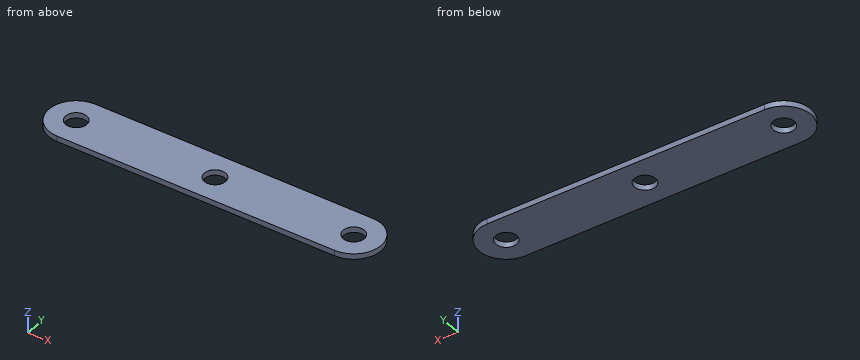
```python
from build123d import *

# Parameters (mm, degrees)
BOSS_EXTRUDE1_DEPTH = 4
CUT_EXTRUDE1_REACH  = 6
SKETCH2_R           = 7.75
CUT_EXTRUDE2_REACH  = 6
SKETCH3_R           = 7.75


with BuildPart() as part:
    # Sketch1 → Boss-Extrude1 (new body)
    with BuildSketch(Plane.XY):
        with BuildLine():
            Line((0, 20), (204, 20))
            ThreePointArc((204, 20), (224, 0), (204, -20))
            Line((204, -20), (0, -20))
            ThreePointArc((0, -20), (-20, 0), (0, 20))
        make_face()
    extrude(amount=BOSS_EXTRUDE1_DEPTH)

    # Sketch2 → Cut-Extrude1 (cut, up to next)
    with BuildSketch(Plane.XY.offset(4), mode=Mode.PRIVATE) as cut_extrude1_sk1:
        Circle(SKETCH2_R)
    cut_extrude1_tool1 = extrude(cut_extrude1_sk1.sketch, amount=-CUT_EXTRUDE1_REACH, mode=Mode.PRIVATE) & part.part
    add(cut_extrude1_tool1.solids().sort_by_distance((0, 0, 4))[0], mode=Mode.SUBTRACT)
    # Sketch2 → Cut-Extrude1 (cut, up to next)
    with BuildSketch(Plane.XY.offset(4), mode=Mode.PRIVATE) as cut_extrude1_sk2:
        with Locations((204, 0)):
            Circle(SKETCH2_R)
    cut_extrude1_tool2 = extrude(cut_extrude1_sk2.sketch, amount=-CUT_EXTRUDE1_REACH, mode=Mode.PRIVATE) & part.part
    add(cut_extrude1_tool2.solids().sort_by_distance((204, 0, 4))[0], mode=Mode.SUBTRACT)

    # Sketch3 → Cut-Extrude2 (cut, up to next)
    with BuildSketch(Plane.XY.offset(4), mode=Mode.PRIVATE) as cut_extrude2_sk1:
        with Locations((102, 0)):
            Circle(SKETCH3_R)
    cut_extrude2_tool1 = extrude(cut_extrude2_sk1.sketch, amount=-CUT_EXTRUDE2_REACH, mode=Mode.PRIVATE) & part.part
    add(cut_extrude2_tool1.solids().sort_by_distance((102, 0, 4))[0], mode=Mode.SUBTRACT)


solid = part.part
```
Geometry check sheet. Reference: the model listing, model coordinates, mm. Give positions to 0.01 mm unless a question says otherwise; leave off trailing zeros. Order: outer loops, then holes, each group sorted by start corner. A loop starts at its lowest first (then second) coordinate and runs counter-clockwise, first axis right, second up. Notation, with made-up numbers: (42, 18) -> (77, 18) arc R16 cw to (77, 27) -> close; hole circle Ø2 at (64.25, 58). An arc over 180 degrees is marked (long way). Write each question's results on one line, items separated by ' | '. Start each with the question number.
(1) Gauge pin test, flat end, axial feed: P1, Ø1, axis at y = 2, z = 2.5, coming from the -X side. Record the tip position at first contact, or that the pin passes through.
(2) Sectioned sample at D-D (y = 12). Enter the section's corners in (x, z), plus the area to 3 significant figures.
(3) Sectioned sample at A-A (y = 0). Enter the section's corners in (x, z).
(4) Sectioned sample at B-B (z = 2.45). Enter the section's corners in (x, y), plus the area to 3 significant figures.
(5) Scan lines: line 1 (Y direction, x = 0, z = 3.15); line 2 (X direction, y = 4, z = 0.3); line 3 (Y direction, x = 104.5, z = 1.95). Record each from-to range of solid material in increasing order.
(6) Sectioned sample at C-C (x = 102). Enter the section's corners in (y, z).
Answer below:
1) P1: x = -19.94
2) outline: (-16, 0) -> (220, 0) -> (220, 4) -> (-16, 4) -> close | area: 944 mm2
3) outline: (-20, 0) -> (-7.75, 0) -> (-7.75, 4) -> (-20, 4) -> close; (7.75, 0) -> (94.25, 0) -> (94.25, 4) -> (7.75, 4) -> close; (109.75, 0) -> (196.25, 0) -> (196.25, 4) -> (109.75, 4) -> close; (211.75, 0) -> (224, 0) -> (224, 4) -> (211.75, 4) -> close
4) outline: (0, -20) -> (204, -20) arc R20 ccw to (204, 20) -> (0, 20) arc R20 ccw to start; hole circle Ø15.5 at (0, 0); hole circle Ø15.5 at (102, 0); hole circle Ø15.5 at (204, 0) | area: 8,850 mm2
5) line 1: -20 to -7.75, 7.75 to 20 | line 2: -19.6 to -6.64, 6.64 to 95.36, 108.64 to 197.36, 210.64 to 223.6 | line 3: -20 to -7.34, 7.34 to 20
6) outline: (-20, 0) -> (-7.75, 0) -> (-7.75, 4) -> (-20, 4) -> close; (7.75, 0) -> (20, 0) -> (20, 4) -> (7.75, 4) -> close
